from build123d import *

# Parameters (mm, degrees)
SKETCH1_W           = 120
SKETCH1_H           = 120
BOSS_EXTRUDE1_DEPTH = 3
CAVITY1_DEPTH       = 3
SKETCH5_R           = 1.5
CUT_EXTRUDE3_DEPTH  = 3
SKETCH6_R           = 1.5
CUT_EXTRUDE4_DEPTH  = 3
SKETCH8_R           = 1.5
CUT_EXTRUDE6_DEPTH  = 3


# Read off the part's stored shape, not the designer's step: Cavity1
with BuildPart() as part:
    # Sketch1 → Boss-Extrude1 (new body)
    with BuildSketch(Plane(origin=(0, 0, 0), x_dir=(1, 0, 0), z_dir=(0, 1, 0))):
        with Locations((60, -60)):
            Rectangle(SKETCH1_W, SKETCH1_H)
    extrude(amount=BOSS_EXTRUDE1_DEPTH)

    # Cavity1 outline → Cavity1 (cut)
    with BuildSketch(Plane(origin=(0, 0, 0), x_dir=(1, 0, 0), z_dir=(0, 1, 0))):
        with BuildLine():
            Line((46.211417874, -60.353557562), (59.646450781, -73.78858234))
            ThreePointArc((59.646450781, -73.78858234), (60.000004216, -73.935028843), (60.353557562, -73.788582126))
            Line((60.353557562, -73.788582126), (88.213556312, -45.928566518))
            ThreePointArc((88.213556312, -45.928566518), (88.360002815, -45.575013083), (88.213556098, -45.221459737))
            Line((88.213556098, -45.221459737), (74.778523191, -31.786434959))
            ThreePointArc((74.778523191, -31.786434959), (74.424969756, -31.639988457), (74.07141641, -31.786435173))
            Line((74.07141641, -31.786435173), (46.21141766, -59.646450781))
            ThreePointArc((46.21141766, -59.646450781), (46.064971157, -60.000004216), (46.211417874, -60.353557562))
        make_face()
    extrude(amount=CAVITY1_DEPTH, mode=Mode.SUBTRACT)

    # Sketch5 → Cut-Extrude3 (cut)
    with BuildSketch(Plane(origin=(0, 3, 0), x_dir=(1, 0, 0), z_dir=(0, 1, 0))):
        with Locations(Location((60, -10, 0), (0, 0, 270))):
            Circle(SKETCH5_R)
        with Locations(Location((95.355339059, -24.644660941, 0), (0, 0, 270))):
            Circle(SKETCH5_R)
        with Locations(Location((110, -60, 0), (0, 0, 270))):
            Circle(SKETCH5_R)
        with Locations(Location((95.355339059, -95.355339059, 0), (0, 0, 270))):
            Circle(SKETCH5_R)
        with Locations(Location((60, -110, 0), (0, 0, 270))):
            Circle(SKETCH5_R)
        with Locations(Location((24.644660941, -95.355339059, 0), (0, 0, 270))):
            Circle(SKETCH5_R)
        with Locations(Location((10, -60, 0), (0, 0, 270))):
            Circle(SKETCH5_R)
        with Locations(Location((24.644660941, -24.644660941, 0), (0, 0, 270))):
            Circle(SKETCH5_R)
    extrude(amount=-CUT_EXTRUDE3_DEPTH, mode=Mode.SUBTRACT)

    # Sketch6 → Cut-Extrude4 (cut)
    with BuildSketch(Plane(origin=(0, 3, 0), x_dir=(1, 0, 0), z_dir=(0, 1, 0))):
        with Locations(Location((10, -10, 0), (0, 0, 270))):
            Circle(SKETCH6_R)
        with Locations(Location((110, -10, 0), (0, 0, 270))):
            Circle(SKETCH6_R)
        with Locations(Location((110, -110, 0), (0, 0, 270))):
            Circle(SKETCH6_R)
        with Locations(Location((10, -110, 0), (0, 0, 270))):
            Circle(SKETCH6_R)
    extrude(amount=-CUT_EXTRUDE4_DEPTH, mode=Mode.SUBTRACT)

    # Sketch8 → Cut-Extrude6 (cut)
    with BuildSketch(Plane(origin=(0, 3, 0), x_dir=(1, 0, 0), z_dir=(0, 1, 0))):
        with Locations(Location((87.994675608, -39.154311265, 0), (0, 0, 270))):
            Circle(SKETCH8_R)
        with Locations(Location((80.923607796, -32.083243453, 0), (0, 0, 270))):
            Circle(SKETCH8_R)
        with Locations(Location((46.416796874, -66.590054375, 0), (0, 0, 270))):
            Circle(SKETCH8_R)
        with Locations(Location((53.487864686, -73.661122187, 0), (0, 0, 270))):
            Circle(SKETCH8_R)
    extrude(amount=-CUT_EXTRUDE6_DEPTH, mode=Mode.SUBTRACT)


solid = part.part
Design review of the part built by this model. Coordinates are the model's own, in mm. A direction names the side the tool comes from. Coordinates: 2 decimals unless noted, no trailing zeros. Order: outer loops, then holes, each group sorted by start corner. A loop starts at its lowest first (then second) coordinate and runs counter-clockwise, first axis right, second up. Notation, with made-up numbers: (-26.5, 35.25) -> (5.5, 35.25) arc R23 ccw to (5.5, 45.25) -> close; hole circle Ø4 at (-27, 8). An arc over 180 degrees is marked (long way). Use one line per item in the form item = value. Start each with the question number.
(1) Insertion check: pin 1 (2.5 mm diameter, centred on x = 80.92, z = 32.08, fed in from -Y). The pin has a flat end and moves straight along its axis. Give the tip position at first contact, or say it passes through.
(2) For faces 3 (the flat face through (46, 0, 59)), 4 (the flat face through (60.34, 1.48, 45.52)), list the 3-axis set-ups (+Z, -Z, +X, -X, +Y, -Y) from which the entire face can be reached by the end or side of a thin tool; tool diameter is ignored.
(3) For probe 1 along Z at (x, y) = (110, 0.75); probe 2 along Z at (x, y) = (61, 0.4); probe 3 along Z at (x, y) = (25.5, 0.65), list the stretches that pass through material, from the lowest coordinate up.
(4) Add section D-D on x = 63. State the section outline as (y, z) points.
(5) Add section B-B on x = 10. State the section outline as (y, z) points.
(6) The part is to be moulded in two halves that separate along X. For faces 1 (the cylindrical face through (60.07, 1.52, 108.5)), 2 (the flat face through (59, 1, 0)), say which applies: +X half, -X half, draft (parallel to the pull), parting line (faces both ways), or undercut.
(7) Add section C-C on z = 50.5. State the section outline as (x, y) points.
(8) Add section A-A on z = 110. State the section outline as (x, y) points.
Answer block:
q1.pin_1 = through
q2.face_3 = +Z, -Z, +X, -X, -Y
q2.face_4 = +Y, -Y
q3.probe_1 = 0 to 8.5, 11.5 to 58.5, 61.5 to 108.5, 111.5 to 120
q3.probe_2 = 0 to 8.88, 11.12 to 44.86, 73.14 to 108.88, 111.12 to 120
q3.probe_3 = 0 to 23.41, 25.88 to 94.12, 96.59 to 120
q4.outline = (0, 0) -> (3, 0) -> (3, 42.86) -> (0, 42.86) -> close; (0, 71.14) -> (3, 71.14) -> (3, 120) -> (0, 120) -> close
q5.outline = (0, 0) -> (3, 0) -> (3, 8.5) -> (0, 8.5) -> close; (0, 11.5) -> (3, 11.5) -> (3, 58.5) -> (0, 58.5) -> close; (0, 61.5) -> (3, 61.5) -> (3, 108.5) -> (0, 108.5) -> close; (0, 111.5) -> (3, 111.5) -> (3, 120) -> (0, 120) -> close
q6.face_1 = undercut
q6.face_2 = draft
q7.outline = (0, 0) -> (55.36, 0) -> (55.36, 3) -> (0, 3) -> close; (83.64, 0) -> (120, 0) -> (120, 3) -> (83.64, 3) -> close
q8.outline = (0, 0) -> (8.5, 0) -> (8.5, 3) -> (0, 3) -> close; (11.5, 0) -> (58.5, 0) -> (58.5, 3) -> (11.5, 3) -> close; (61.5, 0) -> (108.5, 0) -> (108.5, 3) -> (61.5, 3) -> close; (111.5, 0) -> (120, 0) -> (120, 3) -> (111.5, 3) -> close
